Could you check a few things on this model? Use its own coordinates, in mm. Face numbers are marked on the shaded views. A direction names the side the tool comes from. Round coordinates to 2 decimals unless told otherwise and drop trailing zeros. Order: outer loops, then holes, each group sorted by start corner. A loop starts at its lowest first (then second) coordinate and runs counter-clockwise, first axis right, second up. Notation, with made-up numbers: (70.25, -23) -> (91.25, -23) arc R26 cw to (91.25, -5) -> close; hole circle Ø11 at (78.5, 64.5). An arc over 180 degrees is marked (long way). Put each result on its own line as item: value. Start each with the question number.
from build123d import *

# Parameters (mm, degrees)
F0_R      = 50.8
F1_DEPTH  = 5.08
F2_R      = 50.2158
F3_DEPTH  = 5.08
F4_R      = 49.1744
F5_DEPTH  = 5.08
F6_R      = 47.5742
F7_DEPTH  = 5.08
F8_R      = 45.3644
F9_DEPTH  = 5.08
F10_R     = 42.291
F11_DEPTH = 5.08
F12_R     = 38.608
F13_DEPTH = 5.08
F14_R     = 33.6042
F15_DEPTH = 5.08
F16_R     = 26.7716
F17_DEPTH = 5.08
F18_R     = 15.8496
F19_DEPTH = 5.08


with BuildPart() as f1:
    # F0 (on Top) → F1 (new body)
    with BuildSketch(Plane.XY):
        Circle(F0_R)
    extrude(amount=F1_DEPTH)

    # F2 (on face) → F3 (join)
    with BuildSketch(Plane.XY.offset(5.08)):
        Circle(F2_R)
    extrude(amount=F3_DEPTH)

    # F4 (on face) → F5 (join)
    with BuildSketch(Plane.XY.offset(10.16)):
        Circle(F4_R)
    extrude(amount=F5_DEPTH)

    # F6 (on face) → F7 (join)
    with BuildSketch(Plane.XY.offset(15.24)):
        Circle(F6_R)
    extrude(amount=F7_DEPTH)

    # F8 (on face) → F9 (join)
    with BuildSketch(Plane.XY.offset(20.32)):
        Circle(F8_R)
    extrude(amount=F9_DEPTH)

    # F10 (on face) → F11 (join)
    with BuildSketch(Plane.XY.offset(25.4)):
        Circle(F10_R)
    extrude(amount=F11_DEPTH)

    # F12 (on face) → F13 (join)
    with BuildSketch(Plane.XY.offset(30.48)):
        Circle(F12_R)
    extrude(amount=F13_DEPTH)

    # F14 (on face) → F15 (join)
    with BuildSketch(Plane.XY.offset(35.56)):
        Circle(F14_R)
    extrude(amount=F15_DEPTH)

    # F16 (on face) → F17 (join)
    with BuildSketch(Plane.XY.offset(40.64)):
        Circle(F16_R)
    extrude(amount=F17_DEPTH)

    # F18 (on face) → F19 (join)
    with BuildSketch(Plane.XY.offset(45.72)):
        Circle(F18_R)
    extrude(amount=F19_DEPTH)


solid = f1.part
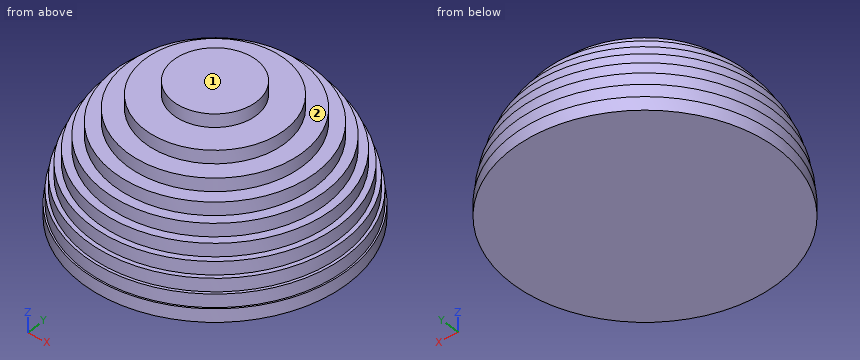
1. For pin 1 Ø12 at (x, z) = (-21, 43) entering from -Y; pin 2 Ø5 at (y, z) = (34.5, 11.5) entering from +X; pin 3 Ø1.5 at (x, z) = (15, 7) entering from +Y, each with a flat end and sliding along its axis, tell me the tip position at first contact or that it passes through.
2. If we section it at A-A, the plane x = -40: Please give me the cut outline in (y, z).
3. If we section it at C-C, the plane y = -44: Please give me the cut outline in (x, z), then the cut area to 3 significant figures.
4. Which directions (+Z, -Z, +X, -X, +Y, -Y) give clear straight access to the entire face, cutting with the end or side of a thin tool? Please do the marked faces 1 and 2.
5. I need wall thicknesses on L1, parallel to Y at x = -1, z = 14; L2, parallel to Z at x = -18.5, y = 22; L3, parallel to X at y = -37, z = 12.5. Which ranges of each line are inside material? Lowest first, please.
Results below:
1. pin 1: y = -29.82
1. pin 2: x = 38.37
1. pin 3: y = 48.15
2. outline: (-31.32, 0) -> (31.32, 0) -> (31.32, 5.08) -> (30.36, 5.08) -> (30.36, 10.16) -> (28.6, 10.16) -> (28.6, 15.24) -> (25.75, 15.24) -> (25.75, 20.32) -> (21.4, 20.32) -> (21.4, 25.4) -> (13.73, 25.4) -> (13.73, 30.48) -> (-13.73, 30.48) -> (-13.73, 25.4) -> (-21.4, 25.4) -> (-21.4, 20.32) -> (-25.75, 20.32) -> (-25.75, 15.24) -> (-28.6, 15.24) -> (-28.6, 10.16) -> (-30.36, 10.16) -> (-30.36, 5.08) -> (-31.32, 5.08) -> close
3. outline: (-25.39, 0) -> (25.39, 0) -> (25.39, 5.08) -> (24.2, 5.08) -> (24.2, 10.16) -> (21.96, 10.16) -> (21.96, 15.24) -> (18.09, 15.24) -> (18.09, 20.32) -> (11.04, 20.32) -> (11.04, 25.4) -> (-11.04, 25.4) -> (-11.04, 20.32) -> (-18.09, 20.32) -> (-18.09, 15.24) -> (-21.96, 15.24) -> (-21.96, 10.16) -> (-24.2, 10.16) -> (-24.2, 5.08) -> (-25.39, 5.08) -> close
3. area: 1,020 mm2
4. face 1: +Z, +X, -X, +Y, -Y
4. face 2: +Z
5. L1: -49.16 to 49.16
5. L2: 0 to 40.64
5. L3: -32.39 to 32.39
